```python
from build123d import *

# Parameters (mm, degrees)
SKETCH1_R                = 60
SKETCH1_R_2              = 45
SKETCH1_R_3              = 42.5
SKETCH1_R_4              = 2
BOSS_EXTRUDE1_DEPTH      = 1.25
BOSS_EXTRUDE1_DEPTH_BACK = 1.25
SKETCH1_3_R              = 45
SKETCH1_3_R_2            = 42.5
SKETCH1_3_R_3            = 2
BOSS_EXTRUDE2_DEPTH      = 11.75
SKETCH1_4_R              = 62.5
SKETCH1_4_R_2            = 60
BOSS_EXTRUDE3_DEPTH      = 15
BOSS_EXTRUDE3_DEPTH_BACK = 1.25


with BuildPart() as part:
    # Sketch1 → Boss-Extrude1 (new, two sides)
    with BuildSketch(Plane.XY) as boss_extrude1_sk:
        Circle(SKETCH1_R)
        Circle(SKETCH1_R_2, mode=Mode.SUBTRACT)
        with BuildLine():
            ThreePointArc((-45.033320997, -26), (-42.301270189, -26.732050808), (-41.569219382, -24))
            ThreePointArc((-41.569219382, -24), (-46.364439662, 12.423314165), (-24, 41.569219382))
            ThreePointArc((-24, 41.569219382), (-23.267949192, 44.301270189), (-26, 45.033320997))
            ThreePointArc((-26, 45.033320997), (-50.228142967, 13.458590345), (-45.033320997, -26))
        make_face(mode=Mode.SUBTRACT)
        with BuildLine():
            ThreePointArc((45.033320997, -26), (44.301270189, -23.267949192), (41.569219382, -24))
            ThreePointArc((41.569219382, -24), (12.423314165, -46.364439662), (-24, -41.569219382))
            ThreePointArc((-24, -41.569219382), (-26.732050808, -42.301270189), (-26, -45.033320997))
            ThreePointArc((-26, -45.033320997), (13.458590345, -50.228142967), (45.033320997, -26))
        make_face(mode=Mode.SUBTRACT)
        with BuildLine():
            ThreePointArc((0, 52), (-2, 50), (0, 48))
            ThreePointArc((0, 48), (33.941125497, 33.941125497), (48, 0))
            ThreePointArc((48, 0), (50, -2), (52, 0))
            ThreePointArc((52, 0), (36.769552622, 36.769552622), (0, 52))
        make_face(mode=Mode.SUBTRACT)
        Circle(SKETCH1_R_2)
        Circle(SKETCH1_R_3, mode=Mode.SUBTRACT)
        Circle(SKETCH1_R_3)
        Circle(SKETCH1_R_4, mode=Mode.SUBTRACT)
        with Locations((14.715815051, -14.981481481)):
            Circle(SKETCH1_R_4, mode=Mode.SUBTRACT)
        with Locations((0, -27)):
            Circle(SKETCH1_R_4, mode=Mode.SUBTRACT)
        with Locations((14.715815051, -14.981481481)):
            Circle(SKETCH1_R_4)
    extrude(amount=BOSS_EXTRUDE1_DEPTH)
    extrude(boss_extrude1_sk.sketch, amount=-BOSS_EXTRUDE1_DEPTH_BACK)

    # Sketch1_3 → Boss-Extrude2 (add)
    with BuildSketch(Plane.XY):
        Circle(SKETCH1_3_R)
        Circle(SKETCH1_3_R_2, mode=Mode.SUBTRACT)
        with Locations((14.715815051, -14.981481481)):
            Circle(SKETCH1_3_R_3)
    extrude(amount=BOSS_EXTRUDE2_DEPTH)

    # Sketch1_4 → Boss-Extrude3 (add, two sides)
    with BuildSketch(Plane.XY) as boss_extrude3_sk:
        Circle(SKETCH1_4_R)
        Circle(SKETCH1_4_R_2, mode=Mode.SUBTRACT)
    extrude(amount=BOSS_EXTRUDE3_DEPTH)
    extrude(boss_extrude3_sk.sketch, amount=-BOSS_EXTRUDE3_DEPTH_BACK)


solid = part.part
```
Part model, mm, in its own coordinate system. A direction names the side the tool comes from. Round coordinates to 2 decimals unless told otherwise and drop trailing zeros. Write each loop counter-clockwise with the first axis right and the second up, starting at its lowest first coordinate (ties: lowest second). Pieces come first, ordered by that corner, then holes. Notation, with made-up numbers: M -3,-6 L 33,-6 A19 cw 33,7 Z; hole C -26.75,-14.5 d8. An arc over 180 degrees is marked long. Answer as CSV lines item,"result". Start each with the question number.
1) Which spindle directions (+Z, -Z, +X, -X, +Y, -Y) get a long thin tool onto all of the face, cutting with end or side? Do faces 3 (the face through (-1, -13, -1.25)), 4 (the face through (20.765, -39.923, 6.426)), 5 (the face through (33.57, 34.31, -0.02)). Say none if no direction does.
2) Drop flat-ended pins along their axis: pin 1 (5 mm diameter, centred on x = 0, y = 0, fed in from +Z); pin 2 (1.5 mm diameter, centred on y = 35, z = 7, fed in from -X); pin 3 (6 mm diameter, centred on x = -38, z = 12, fed in from -Y). Give the stop position or say it passes through.
3) Band-saw the part on A-A (x = 19.5). List the corners of the cut face in (y, z), then the cut area to 3 significant figures.
4) Band-saw the part on C-C (x = 50). List the corners of the cut face in (y, z).
5) Mould opens along X. For faces 1 (the face through (-23, 56, 15)), 2 (the face through (-50.077, 14.01, -0.018)) say: +X half, -X half, draft (parallel to the pull), parting line (faces both ways), or undercut.
6) Band-saw the part on B-B (z = 7.25). List the corners of the cut face in (x, y), then the cut area to 3 significant figures.
7) Band-saw the part on D-D (x = 36.5). List the corners of the cut face in (y, z), then the cut area to 4 significant figures.
8) Drill centre lines: L1, parallel to Y at x = -18, z = 11.5; L2, parallel to X at y = -24.5, z = 9.5; L3, parallel to X at y = 6.5, z = 7.5. Where is each one in solid material? Low to high.
Worked out:
1,face 3,"-Z, +X, -X, +Y, -Y"
1,face 4,"+Z"
1,face 5,"+Z, -Z"
2,pin 1,"z = 1.25"
2,pin 2,"x = -52.28"
2,pin 3,"y = -51.78"
3,outline,"M -59.38,-1.25 L -48.21,-1.25 L -48.21,1.25 L -56.74,1.25 L -56.74,15 L -59.38,15 Z; M -43.86,-1.25 L 43.86,-1.25 L 43.86,1.25 L 40.56,1.25 L 40.56,11.75 L 37.76,11.75 L 37.76,1.25 L -37.76,1.25 L -37.76,11.75 L -40.56,11.75 L -40.56,1.25 L -43.86,1.25 Z; M 48.21,-1.25 L 59.38,-1.25 L 59.38,15 L 56.74,15 L 56.74,1.25 L 48.21,1.25 Z"
3,area,"406 mm²"
4,outline,"M -37.5,-1.25 L -2,-1.25 L -2,1.25 L -33.17,1.25 L -33.17,15 L -37.5,15 Z; M 14.28,-1.25 L 37.5,-1.25 L 37.5,15 L 33.17,15 L 33.17,1.25 L 14.28,1.25 Z"
5,face 1,"draft"
5,face 2,"undercut"
6,outline,"C 0,0 d125; C 0,0 d90; C 14.72,-14.98 d4; hole C 0,0 d120; hole C 0,0 d85"
6,area,"1,660 mm²"
7,outline,"M -50.73,-1.25 L -37.04,-1.25 L -37.04,1.25 L -47.62,1.25 L -47.62,15 L -50.73,15 Z; M -31.17,-1.25 L 31.17,-1.25 L 31.17,1.25 L 26.32,1.25 L 26.32,11.75 L 21.77,11.75 L 21.77,1.25 L -21.77,1.25 L -21.77,11.75 L -26.32,11.75 L -26.32,1.25 L -31.17,1.25 Z; M 37.04,-1.25 L 50.73,-1.25 L 50.73,15 L 47.62,15 L 47.62,1.25 L 37.04,1.25 Z"
7,area,"405.5 mm²"
8,L1,"-59.85 to -57.24, -41.24 to -38.5, 38.5 to 41.24, 57.24 to 59.85"
8,L2,"-57.5 to -54.77, -37.75 to -34.73, 34.73 to 37.75, 54.77 to 57.5"
8,L3,"-62.16 to -59.65, -44.53 to -42, 42 to 44.53, 59.65 to 62.16"
